```python
from build123d import *

# Parameters (mm, degrees)
SKETCH_1_W          = 20
SKETCH_1_H          = 20
SKETCH_1_R          = 1
EXTRUDE_2_DEPTH     = 34
SKETCH_2_R          = 8
EXTRUDE_3_DEPTH     = 1.6
SKETCH_3_R          = 2
EXTRUDE_4_DEPTH     = 13.4
CUT_EXTRUDE_START   = -9
CUT_EXTRUDE_1_DEPTH = 9


with BuildPart() as part:
    # 草图1 → 凸台-拉伸2 (new body)
    with BuildSketch(Plane(origin=(0, 0, 0), x_dir=(0, 0, -1), z_dir=(1, 0, 0))):
        with Locations((10, 10)):
            Rectangle(SKETCH_1_W, SKETCH_1_H)
        with Locations((2.3, 2.3)):
            Circle(SKETCH_1_R, mode=Mode.SUBTRACT)
        with Locations((2.3, 17.7)):
            Circle(SKETCH_1_R, mode=Mode.SUBTRACT)
        with Locations((17.7, 17.7)):
            Circle(SKETCH_1_R, mode=Mode.SUBTRACT)
        with Locations((17.7, 2.298566716)):
            Circle(SKETCH_1_R, mode=Mode.SUBTRACT)
    extrude(amount=EXTRUDE_2_DEPTH)

    # 草图2 → 凸台-拉伸3 (add)
    with BuildSketch(Plane(origin=(34, 0, 0), x_dir=(0, 0, -1), z_dir=(1, 0, 0))):
        with Locations((10, 10)):
            Circle(SKETCH_2_R)
    extrude(amount=EXTRUDE_3_DEPTH)

    # 草图3 → 凸台-拉伸4 (add)
    with BuildSketch(Plane(origin=(35.6, 0, 0), x_dir=(0, 0, -1), z_dir=(1, 0, 0))):
        with Locations((10, 10)):
            Circle(SKETCH_3_R)
    extrude(amount=EXTRUDE_4_DEPTH)

    # 草图4 → 切除-拉伸1 (cut)
    with BuildSketch(Plane(origin=(49, 0, 0), x_dir=(0, 0, -1), z_dir=(1, 0, 0)).offset(CUT_EXTRUDE_START)):
        with BuildLine():
            Line((11.5, 11.322875656), (11.5, 10))
            Line((11.5, 10), (11.5, 8.677124344))
            ThreePointArc((11.5, 8.677124344), (11.870828693, 9.292893219), (12, 10))
            ThreePointArc((12, 10), (11.870828693, 10.707106781), (11.5, 11.322875656))
        make_face()
    extrude(amount=CUT_EXTRUDE_1_DEPTH, mode=Mode.SUBTRACT)


solid = part.part
```
Check sheet for the modelled part. Datum: model origin and axes. Units: mm. A direction names the side the tool comes from. Give positions to 0.01 mm unless a question says otherwise; leave off trailing zeros. Order: outer loops, then holes, each group sorted by start corner. A loop starts at its lowest first (then second) coordinate and runs counter-clockwise, first axis right, second up. Notation, with made-up numbers: M 80.25,45.5 L 123.25,45.5 A34 ccw 123.25,84.5 Z; hole C 5.5,-0.75 d3. An arc over 180 degrees is marked long. Answer in a Markdown table with one row per item.
1) Release check for a two-part mould opening along Y. For faces 4 (the flat face through (17, 0, -10)), 5 (the cylindrical face through (16.8, 17.1, -16.9)), 6 (the flat face through (34, 17, -5)), 7 (the cylindrical face through (16.76, 1.41, -2.76)) record: +Y half, -Y half, draft (parallel to the pull), parting line (faces both ways), or undercut.
Filled sheet:
| item | result |
|---|---|
| face 4 | -Y half |
| face 5 | undercut |
| face 6 | draft |
| face 7 | undercut |
2) Cross-section at B-B, the plane z = -10. Enter the section's corners in (x, y).
Filled sheet:
| item | result |
|---|---|
| outline | M 0,0 L 34,0 L 34,2 L 35.6,2 L 35.6,8 L 49,8 L 49,12 L 35.6,12 L 35.6,18 L 34,18 L 34,20 L 0,20 Z |
3) Cross-section at A-A, the plane y = 10. Enter the section's corners in (x, z), plus the area to 3 significant figures.
Filled sheet:
| item | result |
|---|---|
| outline | M 0,-20 L 34,-20 L 34,-18 L 35.6,-18 L 35.6,-12 L 40,-12 L 40,-11.5 L 49,-11.5 L 49,-8 L 35.6,-8 L 35.6,-2 L 34,-2 L 34,0 L 0,0 Z |
| area | 755 mm2 |
4) Cross-section at C-C, the plane x = 4.5. Enter the section's corners in (y, z).
Filled sheet:
| item | result |
|---|---|
| outline | M 0,-20 L 20,-20 L 20,0 L 0,0 Z; hole C 2.3,-17.7 d2; hole C 2.3,-2.3 d2; hole C 17.7,-17.7 d2; hole C 17.7,-2.3 d2 |
5) Access from +Z, -Z, +X, -X, +Y, -Y to the whole of each face (thin tool, end or side, straight path). Record for faces 1 (the cylindrical face through (34.79, 2.19, -8.27)), 2 (the flat face through (49, 10, -10)), 3 (the flat face through (44, 10, -11.5)).
Filled sheet:
| item | result |
|---|---|
| face 1 | +X |
| face 2 | +Z, -Z, +X, +Y, -Y |
| face 3 | -Z, +X, +Y, -Y |
6) Gauge pin test, flat ends, axial feed: P1, Ø4, axis at y = 8, z = -4, coming from the +X side; P2, Ø2, axis at x = 42.5, y = 10.5, coming from the -Z side. Record the tip position at first contact, or that the pin passes through.
Filled sheet:
| item | result |
|---|---|
| P1 | stops at x = 35.6 |
| P2 | stops at z = -11.5 |
7) Thickness scan on L1, parallel to Y at x = 11, z = -17.7; L2, parallel to Z at x = 15.5, y = 17; L3, parallel to Y at x = 28, z = -17.25. Record the ranges inside material, lowest first. Write a range as [from, to].
Filled sheet:
| item | result |
|---|---|
| L1 | y = [0, 1.3], [3.3, 16.7], [18.7, 20] |
| L2 | z = [-20, -18.41], [-16.99, -3.01], [-1.59, 0] |
| L3 | y = [0, 1.41], [3.19, 16.81], [18.59, 20] |
8) Cross-section at D-D, the plane y = 13.25. Enter the section's corners in (x, z), plus the area to 3 significant figures.
Filled sheet:
| item | result |
|---|---|
| outline | M 0,-20 L 34,-20 L 34,-17.31 L 35.6,-17.31 L 35.6,-2.69 L 34,-2.69 L 34,0 L 0,0 Z |
| area | 703 mm2 |
